Can you work these out from the model? Positions are in its coordinate system, mm. A direction names the side the tool comes from. Coordinates: 2 decimals unless noted, no trailing zeros. Loops run counter-clockwise (first coordinate to the right, second up) from the corner with the lowest first, then second, coordinate; pieces in that order, holes last.
```python
from build123d import *

# Parameters (mm, degrees)
SKETCH_1_R          = 1.4
EXTRUDE_2_DEPTH     = 2
CUT_EXTRUDE_1_REACH = 26.88


with BuildPart() as part:
    # 草图1 → 凸台-拉伸2 (new body)
    with BuildSketch(Plane.XY):
        Polygon((20.737338075, 10.050011688), (20.737338075, 13.600023376), (-20.737338075, 13.600023376), (-20.737338075, 10.050011688), (-20.437338075, 10.050011688), (-20.237338075, 9.850011688), (-20.237338075, 9.250011688), (-20.437338075, 9.050011688), (-20.737338075, 9.050011688), (-20.737338075, 8.550011688), (-20.437338075, 8.550011688), (-20.237338075, 8.350011688), (-20.237338075, 7.750011688), (-20.437338075, 7.550011688), (-20.737338075, 7.550011688), (-20.737338075, 7.050011688), (-20.437338075, 7.050011688), (-20.237338075, 6.850011688), (-20.237338075, 6.250011688), (-20.437338075, 6.050011688), (-20.737338075, 6.050011688), (-20.737338075, 5.550011688), (-20.437338075, 5.550011688), (-20.237338075, 5.350011688), (-20.237338075, 4.750011688), (-20.437338075, 4.550011688), (-20.737338075, 4.550011688), (-20.737338075, 4.050011688), (-20.437338075, 4.050011688), (-20.237338075, 3.850011688), (-20.237338075, 3.250011688), (-20.437338075, 3.050011688), (-20.737338075, 3.050011688), (-20.737338075, 2.550011688), (-20.437338075, 2.550011688), (-20.237338075, 2.350011688), (-20.237338075, 1.750011688), (-20.437338075, 1.550011688), (-20.737338075, 1.550011688), (-20.737338075, 1.050011688), (-20.437338075, 1.050011688), (-20.237338075, 0.850011688), (-20.237338075, 0.250011688), (-20.437338075, 0.050011688), (-20.737338075, 0.050011688), (-20.737338075, -4.5), (20.737338075, -4.5), (20.737338075, 0.050011688), (20.437338075, 0.050011688), (20.237338075, 0.250011688), (20.237338075, 0.850011688), (20.437338075, 1.050011688), (20.737338075, 1.050011688), (20.737338075, 1.550011688), (20.437338075, 1.550011688), (20.237338075, 1.750011688), (20.237338075, 2.350011688), (20.437338075, 2.550011688), (20.737338075, 2.550011688), (20.737338075, 3.050011688), (20.437338075, 3.050011688), (20.237338075, 3.250011688), (20.237338075, 3.850011688), (20.437338075, 4.050011688), (20.737338075, 4.050011688), (20.737338075, 4.550011688), (20.437338075, 4.550011688), (20.237338075, 4.750011688), (20.237338075, 5.350011688), (20.437338075, 5.550011688), (20.737338075, 5.550011688), (20.737338075, 6.050011688), (20.437338075, 6.050011688), (20.237338075, 6.250011688), (20.237338075, 6.850011688), (20.437338075, 7.050011688), (20.737338075, 7.050011688), (20.737338075, 7.550011688), (20.437338075, 7.550011688), (20.237338075, 7.750011688), (20.237338075, 8.350011688), (20.437338075, 8.550011688), (20.737338075, 8.550011688), (20.737338075, 9.050011688), (20.437338075, 9.050011688), (20.237338075, 9.250011688), (20.237338075, 9.850011688), (20.437338075, 10.050011688), align=None)
        with Locations((-18.383061341, 11.500023376)):
            Circle(SKETCH_1_R, mode=Mode.SUBTRACT)
        with Locations((-18.383061341, -2.4)):
            Circle(SKETCH_1_R, mode=Mode.SUBTRACT)
        with Locations((18.383061341, -2.4)):
            Circle(SKETCH_1_R, mode=Mode.SUBTRACT)
        with Locations((18.383061341, 11.500023376)):
            Circle(SKETCH_1_R, mode=Mode.SUBTRACT)
    extrude(amount=EXTRUDE_2_DEPTH)

    # 草图2 → 切除-拉伸1 (cut, up to next)
    with BuildSketch(Plane(origin=(0, 0, 0), x_dir=(-1, 0, 0), z_dir=(0, 0, -1)), mode=Mode.PRIVATE) as cut_extrude_1_sk1:
        with BuildLine():
            Line((2.97, 4.63388738), (-2.97, 4.63388738))
            ThreePointArc((-2.97, 4.63388738), (-4.030660172, 4.194547552), (-4.47, 3.13388738))
            Line((-4.47, 3.13388738), (-4.47, 2.97388738))
            ThreePointArc((-4.47, 2.97388738), (-4.030660172, 1.913227209), (-2.97, 1.47388738))
            Line((-2.97, 1.47388738), (-0.05, 1.47388738))
            Line((-0.05, 1.47388738), (2.97, 1.47388738))
            ThreePointArc((2.97, 1.47388738), (4.030660172, 1.913227209), (4.47, 2.97388738))
            Line((4.47, 2.97388738), (4.47, 3.13388738))
            ThreePointArc((4.47, 3.13388738), (4.030660172, 4.194547552), (2.97, 4.63388738))
        make_face()
    cut_extrude_1_tool1 = extrude(cut_extrude_1_sk1.sketch, amount=-CUT_EXTRUDE_1_REACH, mode=Mode.PRIVATE) & part.part
    add(cut_extrude_1_tool1.solids().sort_by_distance((0, 3.053887, 0))[0], mode=Mode.SUBTRACT)


solid = part.part
```
(1) I want a section at B-B on y = 11. Write out the boundary of the cut face in (x, z).
Check values:
outline: (-20.74, 0) - (-19.69, 0) - (-19.69, 2) - (-20.74, 2) - close; (-17.08, 0) - (17.08, 0) - (17.08, 2) - (-17.08, 2) - close; (19.69, 0) - (20.74, 0) - (20.74, 2) - (19.69, 2) - close
(2) If we mould it in two halves opening along X, with no side actions, what happens to faces 1 (the flat face through (0, 4.634, 1)), 2 (the flat face through (20.737, -2, 1)), 3 (the flat face through (0, -4.5, 1))? For each: released by +X, released by -X, zero draft, split by the parting line, or undercut.
Check values:
face 1: undercut
face 2: released by +X
face 3: zero draft
(3) I want a section at A-A on y = -2.4. Write out the boundary of the cut face in (x, z).
Check values:
outline: (-20.74, 0) - (-19.78, 0) - (-19.78, 2) - (-20.74, 2) - close; (-16.98, 0) - (16.98, 0) - (16.98, 2) - (-16.98, 2) - close; (19.78, 0) - (20.74, 0) - (20.74, 2) - (19.78, 2) - close
(4) I want a section at C-C on z = 0.5. State how many separate pieces and enclosed holes the cut face has, then the cut area to 3 significant figures.
Check values:
separate pieces: 1
enclosed holes: 5
area: 693 mm2
(5) If I drill on probe 1 along Y at (x, z) = (1.5, 0.1); probe 2 along X at (y, z) = (-3.5, 0.6); probe 3 along X at (y, z) = (12.5, 0.3), over which ranges is the centre line in solid material (lowest first)?
Check values:
probe 1: y = -4.5 to 1.47, 4.63 to 13.6
probe 2: x = -20.74 to -19.25, -17.52 to 17.52, 19.25 to 20.74
probe 3: x = -20.74 to -19.36, -17.4 to 17.4, 19.36 to 20.74
(6) Which directions (+Z, -Z, +X, -X, +Y, -Y) give clear straight access to the entire face, cutting with the end or side of a thin tool? Please do faces 4 (the cylindrical face through (4.04, 1.92, 0.99)), 5 (the flat face through (0, 5, 0)).
Check values:
face 4: +Z, -Z
face 5: -Z, +X, -X, +Y, -Y
